Here's how the part is built. I have some questions about the finished solid (model axes, mm). A direction names the side the tool comes from. Give positions to 0.01 mm unless a question says otherwise; leave off trailing zeros. Loops run counter-clockwise (first coordinate to the right, second up) from the corner with the lowest first, then second, coordinate; pieces in that order, holes last. Notation, with made-up numbers: (88.5, 72.25) - (94.5, 72.25) arc R27 ccw to (94.5, 104.25) - close; hole circle Ø9 at (59, 42). An arc over 180 degrees is marked (long way). Return JSON: item names as keys, results as strings. Group by question number.
(1) If we mould it in two halves opening along Y, with no side actions, what happens to faces 1 (the flat face through (21, 44.332, 7)), 2 (the flat face through (49, 29.204, 5)), 3 (the flat face through (5.757, 49.444, 3.851))? For each: released by +Y, released by -Y, zero draft, split by the parting line, or undercut.
(2) If we section it at C-C (y = 41.25): Please give me the cut outline in (x, z), then the cut area to 3 significant figures.
(3) I need wall thicknesses on probe 1 along Y at (x, z) = (34.5, 5.75); probe 2 along X at (y, z) = (43, 6.75); probe 3 along Y at (x, z) = (53.5, 6.5). Which ranges of each line are inside material? Lowest first, please. Write a range as [from, to].
(4) On a 3-axis mill with a long thin cutter (end or side, diameter ignored), from which of +Z, -Z, +X, -X, +Y, -Y can I reach the whole of each face in a straight line? I mean faces 4 (the flat face through (7, 47, 0.7)), 5 (the flat face through (49, 49, 6)), 6 (the flat face through (11.029, 30, 3)), 7 (the flat face through (25.069, 39, 7)), 8 (the flat face through (63.523, 39, 7)). Say none if no direction works.
(5) For P1, Ø1.6, axis at x = 7.5, y = 30, coming from the -Z side; P2, Ø1.1, axis at x = 43.5, z = 5, coming from the -Y side; P3, Ø4, axis at x = 21, y = 37.5, coming from the -Z side, each with a flat end and sliding along its axis, tell me the tip position at first contact or that it passes through.
(6) If we section it at D-D (x = 29.5): Please give me the cut outline in (y, z).
(7) If we section it at B-B (y = 37): Please give me the cut outline in (x, z), then the cut area to 3 significant figures.
(8) If we section it at A-A (x = 53): Please give me the cut outline in (y, z).
```python
from build123d import *

# Parameters (mm, degrees)
BOSS_EXTRUDE2_DEPTH       = 7.7
BOSS_EXTRUDE3_DEPTH       = 58.493998982
BOSS_EXTRUDE4_REACH       = 69.972
SKETCH7_W                 = 6
SKETCH7_H                 = 7
BOSS_EXTRUDE5_DEPTH       = 1.9
SKETCH9_W                 = 5
SKETCH9_H                 = 0.4
CUT_EXTRUDE1_DEPTH        = 6
SKETCH10_W                = 51.633694728
SKETCH10_H                = 3.1
BOSS_EXTRUDE6_DEPTH       = 1
MIRROR1_START             = 27.403764687
MIRROR1_DEPTH             = 2.800044537
MIRROR1_START_2           = 29.203809224
MIRROR1_2_DEPTH           = 1
MIRROR1_START_3           = 30.203809224
MIRROR1_3_OUTLINE_W       = 6
MIRROR1_3_OUTLINE_H       = 7
MIRROR1_3_DEPTH           = 0.9
MIRROR1_4_OUTLINE_W       = 0.860304254
MIRROR1_4_OUTLINE_H       = 3.1
MIRROR1_4_DEPTH           = 1.800044537
MIRROR1_START_4           = 5.029168405
MIRROR1_5_OUTLINE_W       = 1
MIRROR1_5_OUTLINE_H       = 3.9
MIRROR1_5_DEPTH           = 6
BOSS_EXTRUDE7_START       = -1.7
BOSS_EXTRUDE7_DEPTH       = 1.7
BOSS_EXTRUDE12_DEPTH      = 3
BOSS_EXTRUDE12_DEPTH_BACK = 1.7
SKETCH14_W                = 1.4
SKETCH14_H                = 19.327817751
FILLET1_R                 = 2
CUT_EXTRUDE2_DEPTH        = 0.6
CUT_EXTRUDE3_DEPTH        = 1.7
SKETCH18_W                = 2
SKETCH18_H                = 2.1
BOSS_EXTRUDE13_DEPTH      = 5.3
SKETCH19_W                = 9.243692919
SKETCH19_H                = 7.158225614
CUT_EXTRUDE4_DEPTH        = 1.7
SKETCH20_W                = 4.7
SKETCH20_H                = 7.158225614
CUT_EXTRUDE5_DEPTH        = 1.4
SKETCH21_W                = 2
SKETCH21_H                = 10.927906825
CUT_EXTRUDE6_DEPTH        = 84.772901086


with BuildPart() as part:
    # Sketch1 → Boss-Extrude2 (new body)
    with BuildSketch(Plane.XY):
        with BuildLine():
            Line((1.569168405, 30.881718108), (1.569168405, 46.853718091))
            ThreePointArc((1.569168405, 46.853718091), (2.581495272, 49.306663259), (5.029168405, 50.331671512))
            Line((5.029168405, 50.331671512), (5.029168405, 48.631626975))
            ThreePointArc((5.029168405, 48.631626975), (3.783584613, 48.104573798), (3.269168405, 46.853718091))
            Line((3.269168405, 46.853718091), (3.269168405, 30.881718108))
            ThreePointArc((3.269168405, 30.881718108), (3.783584613, 29.630862401), (5.029168405, 29.103809224))
            Line((5.029168405, 29.103809224), (5.029168405, 27.403764687))
            ThreePointArc((5.029168405, 27.403764687), (2.581495272, 28.428772939), (1.569168405, 30.881718108))
        make_face()
    extrude(amount=BOSS_EXTRUDE2_DEPTH)

    # Sketch3 → Boss-Extrude3 (add)
    with BuildSketch(Plane(origin=(5.029168405, 0, 0), x_dir=(0, 0, -1), z_dir=(1, 0, 0))):
        Polygon((-7.7, 48.631626975), (-7.7, 50.331671512), (-6.1, 50.331671512), (-6.1, 48.631626975), (-6.1, 48.531626975), (-7.7, 48.531626975), align=None)
    extrude(amount=BOSS_EXTRUDE3_DEPTH)

    # Boss-Extrude4: up to this face of the body (flat: up to its plane)
    boss_extrude4_end = Plane(part.part.faces().sort_by_distance((34.276167896, 48.531626975, 6.9))[0])
    # Sketch4 → Boss-Extrude4 (add, up to the picked face)
    with BuildSketch(Plane(origin=(0, 50.331671512, 0), x_dir=(1, 0, 0), z_dir=(0, 1, 0)), mode=Mode.PRIVATE) as boss_extrude4_sk1:
        Polygon((35.231704884, -6.1), (5.029168405, -6.1), (5.029168405, -3.123421356), (6.505747049, -4.6), (33.731704884, -4.6), (35.202415562, -6.070710678), align=None)
    boss_extrude4_tool1 = split(extrude(boss_extrude4_sk1.sketch, amount=-BOSS_EXTRUDE4_REACH, mode=Mode.PRIVATE), bisect_by=boss_extrude4_end, keep=Keep.BOTH, mode=Mode.PRIVATE)
    add(boss_extrude4_tool1.solids().sort_by(Axis((19.415766, 50.331672, 5.326299), (0, -1, 0)))[0])

    # Sketch7 → Boss-Extrude5 (add)
    with BuildSketch(Plane.XZ.offset(-48.531626975)):
        with Locations((8.029168405, 4.2)):
            Rectangle(SKETCH7_W, SKETCH7_H)
    extrude(amount=BOSS_EXTRUDE5_DEPTH)

    # Sketch8 → Cut-Revolve1 (revolve, cut)
    with BuildSketch(Plane(origin=(0, 48.531626975, 0), x_dir=(1, 0, 0), z_dir=(0, 1, 0))):
        with BuildLine():
            Line((7.493162671, -2.25), (9.593162671, -2.25))
            Line((9.593162671, -2.25), (11.029168405, -2.25))
            Line((11.029168405, -2.25), (11.029168405, -3.013237094))
            add(Edge.make_bspline(
                [(11.029168405, -3.013237094), (10.455622255, -2.979221008), (9.952164105, -2.7)],
                knots=[0, 0, 0, 1, 1, 1], degree=2))
            add(Edge.make_bspline(
                [(8.543162671, -3.3), (9.366293549, -3.339525323), (9.952164105, -2.7)],
                knots=[0, 0, 0, 1, 1, 1], degree=2))
            ThreePointArc((8.543162671, -3.3), (7.800700551, -2.99246212), (7.493162671, -2.25))
        make_face()
    revolve(axis=Axis((7.493162671, 48.531626975, 2.25), (1, 0, 0)), mode=Mode.SUBTRACT)

    # Sketch9 → Cut-Extrude1 (cut)
    with BuildSketch(Plane(origin=(11.029168405, 0, 0), x_dir=(0, 0, -1), z_dir=(1, 0, 0))):
        with Locations((-3.2, 48.331626975)):
            Rectangle(SKETCH9_W, SKETCH9_H)
    extrude(amount=-CUT_EXTRUDE1_DEPTH, mode=Mode.SUBTRACT)

    # Sketch10 → Boss-Extrude6 (add)
    with BuildSketch(Plane(origin=(0, 48.531626975, 0), x_dir=(-1, 0, 0), z_dir=(0, -1, 0))):
        with Locations((-37.706320023, -6.15)):
            Rectangle(SKETCH10_W, SKETCH10_H)
    extrude(amount=BOSS_EXTRUDE6_DEPTH)

    # Mirror1: read off the stored shape, not the designer's step
    # Mirror1 outline → Mirror1 (add)
    with BuildSketch(Plane(origin=(0, 0, 0), x_dir=(1, 0, 0), z_dir=(0, 1, 0)).offset(MIRROR1_START)):
        Polygon((63.523167387, -7.7), (63.523167387, -6.1), (35.231704884, -6.1), (33.731704884, -4.6), (11.889472659, -4.6), (11.889472659, -7.7), align=None)
        Polygon((5.029168405, -7.7), (11.029168405, -7.7), (11.029168405, -4.6), (6.505747049, -4.6), (5.029168405, -3.123421356), align=None)
    extrude(amount=MIRROR1_DEPTH)

    # Mirror1 2 outline → Mirror1 2 (add)
    with BuildSketch(Plane(origin=(0, 0, 0), x_dir=(1, 0, 0), z_dir=(0, 1, 0)).offset(MIRROR1_START_2)):
        Polygon((35.231704884, -6.1), (63.523167387, -6.1), (63.523167387, -4.6), (33.731704884, -4.6), align=None)
    extrude(amount=MIRROR1_2_DEPTH)

    # Mirror1 3 outline → Mirror1 3 (add)
    with BuildSketch(Plane(origin=(0, 0, 0), x_dir=(1, 0, 0), z_dir=(0, 1, 0)).offset(MIRROR1_START_3)):
        with Locations((8.029168405, -4.2)):
            Rectangle(MIRROR1_3_OUTLINE_W, MIRROR1_3_OUTLINE_H)
    extrude(amount=MIRROR1_3_DEPTH)

    # Mirror1 4 outline → Mirror1 4 (add)
    with BuildSketch(Plane(origin=(0, 0, 0), x_dir=(1, 0, 0), z_dir=(0, 1, 0)).offset(MIRROR1_START)):
        with Locations((11.459320532, -6.15)):
            Rectangle(MIRROR1_4_OUTLINE_W, MIRROR1_4_OUTLINE_H)
    extrude(amount=MIRROR1_4_DEPTH)

    # Mirror1 5 outline → Mirror1 5 (add)
    with BuildSketch(Plane.YZ.offset(MIRROR1_START_4)):
        with Locations((29.703809224, 2.65)):
            Rectangle(MIRROR1_5_OUTLINE_W, MIRROR1_5_OUTLINE_H)
    extrude(amount=MIRROR1_5_DEPTH)

    # Mirror1 6 outline → Mirror1 6 (revolve, cut)
    with BuildSketch(Plane(origin=(0, 29.203809224, 2.25), x_dir=(0, 1, 0), z_dir=(0, 0, -1))):
        with BuildLine():
            add(Edge.make_bspline(
                [(0.45, 9.952164105), (0.729221008, 10.455622255), (0.763237094, 11.029168405)],
                knots=[0, 0, 0, 1, 1, 1], degree=2))
            Line((0.763237094, 11.029168405), (0, 11.029168505))
            Line((0, 11.029168505), (0, 7.493162671))
            ThreePointArc((0, 7.493162671), (0.74246212, 7.800700551), (1.05, 8.543162671))
            add(Edge.make_bspline(
                [(1.05, 8.543162671), (1.089525323, 9.366293549), (0.45, 9.952164105)],
                knots=[0, 0, 0, 1, 1, 1], degree=2))
        make_face()
    revolve(axis=Axis((0, 29.203809224, 2.25), (1, 0, 0)), mode=Mode.SUBTRACT)

    # Sketch12 → Boss-Extrude7 (add)
    with BuildSketch(Plane.XY.offset(7.7).offset(BOSS_EXTRUDE7_START)):
        with BuildLine():
            Line((63.523167387, 50.331671512), (5.029168405, 50.331671512))
            ThreePointArc((5.029168405, 50.331671512), (2.581495272, 49.306663259), (1.569168405, 46.853718091))
            Line((1.569168405, 46.853718091), (1.569168405, 30.881718108))
            ThreePointArc((1.569168405, 30.881718108), (2.581495272, 28.428772939), (5.029168405, 27.403764687))
            Line((5.029168405, 27.403764687), (63.523167387, 27.403764687))
            Line((63.523167387, 27.403764687), (63.523167387, 50.331671512))
        make_face()
    extrude(amount=BOSS_EXTRUDE7_DEPTH)

    # Sketch14 → Boss-Extrude12 (add, two sides: drawn at the far end of the back side and taken through both)
    with BuildSketch(Plane(origin=(63.523167387, 0, 0), x_dir=(0, 0, -1), z_dir=(1, 0, 0)).offset(-BOSS_EXTRUDE12_DEPTH_BACK)):
        with Locations((-5.3, 38.8677181)):
            Rectangle(SKETCH14_W, SKETCH14_H)
    extrude(amount=BOSS_EXTRUDE12_DEPTH + BOSS_EXTRUDE12_DEPTH_BACK)

    # Fillet1
    fillet1_edges = [part.edges().sort_by_distance(p)[0] for p in [
        (66.523167387, 48.531626975, 5.3),
        (66.523167387, 29.203809224, 5.3),
    ]]
    fillet(fillet1_edges, radius=FILLET1_R)

    # Sketch15 → Cut-Extrude2 (cut)
    with BuildSketch(Plane.XY.offset(6)):
        with BuildLine():
            Line((63.523167387, 29.203809224), (64.523167387, 29.203809224))
            ThreePointArc((64.523167387, 29.203809224), (65.937380949, 29.789595662), (66.523167387, 31.203809224))
            Line((66.523167387, 31.203809224), (66.523167387, 46.531626975))
            ThreePointArc((66.523167387, 46.531626975), (65.937380949, 47.945840537), (64.523167387, 48.531626975))
            Line((64.523167387, 48.531626975), (63.523167387, 48.531626975))
            Line((63.523167387, 48.531626975), (63.523167387, 29.203809224))
        make_face()
    extrude(amount=-CUT_EXTRUDE2_DEPTH, mode=Mode.SUBTRACT)

    # Sketch16 → Cut-Extrude3 (cut)
    with BuildSketch(Plane.ZY.offset(-1.569168405)):
        with BuildLine():
            Line((1.3, 35.692718099), (1.3, 42.042718099))
            ThreePointArc((1.3, 42.042718099), (3.125, 43.867718099), (4.95, 42.042718099))
            Line((4.95, 42.042718099), (4.95, 35.692718099))
            ThreePointArc((4.95, 35.692718099), (3.125, 33.867718099), (1.3, 35.692718099))
        make_face()
    extrude(amount=-CUT_EXTRUDE3_DEPTH, mode=Mode.SUBTRACT)

    # Sketch18 → Boss-Extrude13 (add)
    with BuildSketch(Plane(origin=(0, 0, 6), x_dir=(-1, 0, 0), z_dir=(0, 0, -1))):
        with Locations((-4.029168405, 47.681626975)):
            Rectangle(SKETCH18_W, SKETCH18_H)
        with Locations((-4.029168405, 30.053809224)):
            Rectangle(SKETCH18_W, SKETCH18_H)
    extrude(amount=BOSS_EXTRUDE13_DEPTH)

    # Sketch19 → Cut-Extrude4 (cut)
    with BuildSketch(Plane.XY.offset(7.7)):
        with Locations((53.076601752, 36.072643067)):
            Rectangle(SKETCH19_W, SKETCH19_H)
    extrude(amount=-CUT_EXTRUDE4_DEPTH, mode=Mode.SUBTRACT)

    # Sketch20 → Cut-Extrude5 (cut)
    with BuildSketch(Plane(origin=(0, 0, 4.6), x_dir=(-1, 0, 0), z_dir=(0, 0, -1))):
        with Locations((-64.173167387, 36.072643067)):
            Rectangle(SKETCH20_W, SKETCH20_H)
    extrude(amount=-CUT_EXTRUDE5_DEPTH, mode=Mode.SUBTRACT)

    # Sketch21 → Cut-Extrude6 (cut, through all)
    with BuildSketch(Plane.XY.offset(7.7)):
        with Locations((20.569168405, 38.867718099)):
            Rectangle(SKETCH21_W, SKETCH21_H)
        with Locations((24.069168405, 38.867718099)):
            Rectangle(SKETCH21_W, SKETCH21_H)
        with Locations((27.569168405, 38.867718099)):
            Rectangle(SKETCH21_W, SKETCH21_H)
    extrude(amount=-CUT_EXTRUDE6_DEPTH, mode=Mode.SUBTRACT)


solid = part.part
```
Values:
{
 "1": {"face 1": "undercut", "face 2": "released by -Y", "face 3": "zero draft"},
 "2": {"outline": "(1.57, 0) - (3.27, 0) - (3.27, 1.3) - (1.57, 1.3) - close; (1.57, 4.95) - (3.27, 4.95) - (3.27, 6) - (19.57, 6) - (19.57, 7.7) - (1.57, 7.7) - close; (21.57, 6) - (23.07, 6) - (23.07, 7.7) - (21.57, 7.7) - close; (25.07, 6) - (26.57, 6) - (26.57, 7.7) - (25.07, 7.7) - close; (28.57, 6) - (61.82, 6) - (61.82, 4.6) - (66.52, 4.6) - (66.52, 5.4) - (63.52, 5.4) - (63.52, 7.7) - (28.57, 7.7) - close", "area": "104 mm2"},
 "3": {"probe 1": "[27.4, 30.2], [47.53, 50.33]", "probe 2": "[1.57, 19.57], [21.57, 23.07], [25.07, 26.57], [28.57, 63.52]", "probe 3": "[27.4, 32.49], [39.65, 50.33]"},
 "4": {"face 4": "-Z, +X", "face 5": "-Z, +X, +Y", "face 6": "-Z", "face 7": "+Z, -Z", "face 8": "+Z, +X, +Y, -Y"},
 "5": {"P1": "z = 0.7", "P2": "y = 29.2", "P3": "z = 6"},
 "6": {"outline": "(27.4, 4.6) - (30.2, 4.6) - (30.2, 6) - (47.53, 6) - (47.53, 4.6) - (50.33, 4.6) - (50.33, 7.7) - (27.4, 7.7) - close"},
 "7": {"outline": "(1.57, 0) - (3.27, 0) - (3.27, 1.3) - (1.57, 1.3) - close; (1.57, 4.95) - (3.27, 4.95) - (3.27, 6) - (19.57, 6) - (19.57, 7.7) - (1.57, 7.7) - close; (21.57, 6) - (23.07, 6) - (23.07, 7.7) - (21.57, 7.7) - close; (25.07, 6) - (26.57, 6) - (26.57, 7.7) - (25.07, 7.7) - close; (28.57, 6) - (48.45, 6) - (48.45, 7.7) - (28.57, 7.7) - close; (57.7, 6) - (63.52, 6) - (63.52, 7.7) - (57.7, 7.7) - close", "area": "83.4 mm2"},
 "8": {"outline": "(27.4, 6) - (29.2, 6) - (29.2, 4.6) - (30.2, 4.6) - (30.2, 6) - (32.49, 6) - (32.49, 7.7) - (27.4, 7.7) - close; (39.65, 6) - (47.53, 6) - (47.53, 4.6) - (48.53, 4.6) - (48.53, 6) - (50.33, 6) - (50.33, 7.7) - (39.65, 7.7) - close"}
}
